For this review, take the finished solid that the model builds, in its own axes (mm). A direction names the side the tool comes from. Give positions to 0.01 mm unless a question says otherwise; leave off trailing zeros. Write each loop counter-clockwise with the first axis right and the second up, starting at its lowest first coordinate (ties: lowest second). Pieces come first, ordered by that corner, then holes. Notation, with made-up numbers: M 60.25,-32 L 109.25,-32 A18 cw 109.25,-19 Z; hole C 45.25,-37 d11. An arc over 180 degrees is marked long. One line per item, written item: value. Start each with the question number.
Item 1: Consider section A-A, the plane y = 0. Write out the cut boundary in (x, z).
Item 2: Clearance check with flat-ended pins moving along their axes: pin 1 Ø6 at (x, z) = (8, 5.5) entering from +Y; pin 2 Ø1 at (y, z) = (2.5, 15) entering from +X; pin 3 Ø4 at (y, z) = (4, 4) entering from -X. State where each tip first meets the part, or that it passes through.
Item 3: Tool access review of faces 1 (the face through (-2.579, -1.978, 29.79)), 2 (the face through (0, 0, 45)): name each direction out of +Z, -Z, +X, -X, +Y, -Y from which nothing blocks a thin tool from reaching the whole face with its end or side.
Item 4: Consider section B-B, the plane z = -5. Write out the cut boundary in (x, y), and give its area (3 significant figures).
Item 5: Consider section C-C, the plane x = 17. Write out the cut boundary in (y, z), and give its area (3 significant figures).
Item 6: To check wall thickness, follow probe 1 along Z at (x, y) = (5.5, 2.75); probe 2 along Y at (x, z) = (14.5, 12). State the ranges of each line that lie inside material, in increasing order.
Item 7: Consider section D-D, the plane z = 34. Write out the cut boundary in (x, y), and give its area (3 significant figures).
```python
from build123d import *

# Parameters (mm, degrees)
ESBO_O1_R                = 3.25
ESBO_O1_R_2              = 6.35
RESSALTO_EXTRUS_O1_DEPTH = 15
RESSALTO_EXTRUS_O2_DEPTH = 30
ESBO_O1_3_R              = 3.25
RESSALTO_EXTRUS_O3_DEPTH = 45


with BuildPart() as part:
    # Esbo_o1 → Ressalto-extrus_o1 (new body, symmetric)
    with BuildSketch(Plane.XY):
        Circle(ESBO_O1_R)
        Circle(ESBO_O1_R_2)
        Circle(ESBO_O1_R, mode=Mode.SUBTRACT)
    extrude(amount=RESSALTO_EXTRUS_O1_DEPTH, both=True)

    # Esbo_o2 → Ressalto-extrus_o2 (add)
    with BuildSketch(Plane.XY.offset(15)):
        with BuildLine():
            ThreePointArc((5.455272679, -3.25), (3.137275888, -5.520869497), (0, -6.35))
            Line((0, -6.35), (20, -6.35))
            Line((20, -6.35), (20, -3.25))
            Line((20, -3.25), (5.455272679, -3.25))
        make_face()
        with BuildLine():
            ThreePointArc((6.35, 0), (-4.490128061, 4.490128061), (0, -6.35))
            Line((0, -6.35), (0, -3.25))
            Line((0, -3.25), (5.455272679, -3.25))
            ThreePointArc((5.455272679, -3.25), (6.122233314, -1.685455204), (6.35, 0))
        make_face()
        with BuildLine():
            Line((0, -3.25), (0, -6.35))
            ThreePointArc((0, -6.35), (3.137275888, -5.520869497), (5.455272679, -3.25))
            Line((5.455272679, -3.25), (0, -3.25))
        make_face()
    extrude(amount=-RESSALTO_EXTRUS_O2_DEPTH)

    # Esbo_o1_3 → Ressalto-extrus_o3 (add)
    with BuildSketch(Plane.XY):
        Circle(ESBO_O1_3_R)
    extrude(amount=RESSALTO_EXTRUS_O3_DEPTH)


solid = part.part
```
Model answer:
1. outline: M -6.35,-15 L 6.35,-15 L 6.35,15 L 3.25,15 L 3.25,45 L -3.25,45 L -3.25,15 L -6.35,15 Z
2. pin 1: stops at y = 3.91
2. pin 2: stops at x = 6.03
2. pin 3: stops at x = -6.03
3. face 1: +Z
3. face 2: +Z, +X, -X, +Y, -Y
4. outline: M 0,-6.35 L 20,-6.35 L 20,-3.25 L 5.46,-3.25 A6.35 ccw long Z
4. area: 177 mm2
5. outline: M -6.35,-15 L -3.25,-15 L -3.25,15 L -6.35,15 Z
5. area: 93.0 mm2
6. probe 1: z = -15 to 15
6. probe 2: y = -6.35 to -3.25
7. outline: C 0,0 d6.5
7. area: 33.2 mm2
